Here's the drawing with two shaded views (mm, measured from the low corner). I have some questions. A direction names the side the tool comes from. Coordinates: 2 decimals unless noted, no trailing zeros. Write each loop counter-clockwise with the first axis right and the second up, starting at its lowest first coordinate (ties: lowest second). Pieces come first, ordered by that corner, then holes.
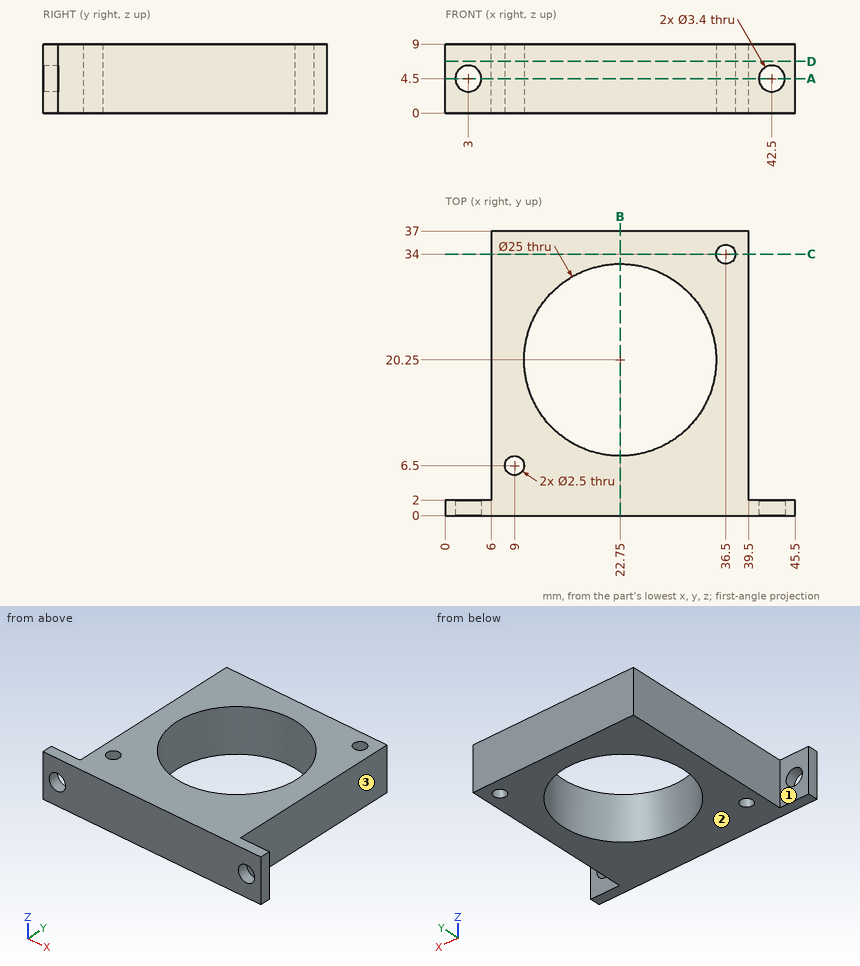
1. I want a section at D-D on z = 6.75. Please give me the cut outline in (x, y), plus the area to 3 significant figures.
Verdict:
outline: (0, 0) - (45.5, 0) - (45.5, 2) - (39.5, 2) - (39.5, 37) - (6, 37) - (6, 2) - (0, 2) - close; hole circle Ø2.5 at (9, 6.5); hole circle Ø25 at (22.75, 20.25); hole circle Ø2.5 at (36.5, 34)
area: 763 mm2
2. I want a section at A-A on z = 4.5. Please give me the cut outline in (x, y), plus the area to 3 significant figures.
Verdict:
outline: (0, 0) - (1.3, 0) - (1.3, 2) - (0, 2) - close; (4.7, 0) - (40.8, 0) - (40.8, 2) - (39.5, 2) - (39.5, 37) - (6, 37) - (6, 2) - (4.7, 2) - close; (44.2, 0) - (45.5, 0) - (45.5, 2) - (44.2, 2) - close; hole circle Ø2.5 at (9, 6.5); hole circle Ø25 at (22.75, 20.25); hole circle Ø2.5 at (36.5, 34)
area: 749 mm2
3. For pin 1 (2.5 mm diameter, centred on y = 26.5, z = 5, fed in from +X); pin 2 (1.8 mm diameter, centred on x = 2.5, z = 3.5, fed in from +Y); pin 3 (5 mm diameter, centred on x = 15.5, y = 26.5, fed in from -Z); pin 4 (2.5 mm diameter, centred on y = 14.5, z = 4, fed in from -X), each with a flat end and sliding along its axis, tell me the tip position at first contact or that it passes through.
Verdict:
pin 1: stops at x = 39.5
pin 2: stops at y = 2
pin 3: passes through
pin 4: stops at x = 6
4. I want a section at C-C on y = 34. Please give me the cut outline in (x, z).
Verdict:
outline: (6, 0) - (35.25, 0) - (35.25, 9) - (6, 9) - close; (37.75, 0) - (39.5, 0) - (39.5, 9) - (37.75, 9) - close
5. Please list where these lines run through material, in increasing order: line 1 along X through (y, z) = (0.9, 4.5); line 2 along Y through (x, z) = (36.5, 6); line 3 along Y through (x, z) = (9, 3.5).
Verdict:
line 1: x = 0 to 1.3, 4.7 to 40.8, 44.2 to 45.5
line 2: y = 0 to 32.75, 35.25 to 37
line 3: y = 0 to 5.25, 7.75 to 37
6. I want a section at B-B on x = 22.75. Please give me the cut outline in (y, z), plus the area to 3 significant figures.
Verdict:
outline: (0, 0) - (7.75, 0) - (7.75, 9) - (0, 9) - close; (32.75, 0) - (37, 0) - (37, 9) - (32.75, 9) - close
area: 108 mm2
7. On a 3-axis mill with a long thin cutter (end or side, diameter ignored), from which of +Z, -Z, +X, -X, +Y, -Y can I reach the whole of each face in a straight line? I mean the marked faces 1, 2 and 3. Say none if no direction works.
Verdict:
face 1: +Z, -Z, -X, +Y
face 2: -Z, +X, -X, +Y, -Y
face 3: +Z, -Z, +X, +Y
